For this review, take the finished solid that the model builds, in its own axes (mm). Face numbers are marked on the shaded views. A direction names the side the tool comes from. Round coordinates to 2 decimals unless told otherwise and drop trailing zeros. Write each loop counter-clockwise with the first axis right and the second up, starting at its lowest first coordinate (ties: lowest second). Pieces come first, ordered by that corner, then holes. Notation, with made-up numbers: M -6.75,-25 L 20.25,-25 A19 ccw 20.25,8 Z; hole C -31,-24 d3. An arc over 180 degrees is marked long. Answer in a Markdown table with one row per item.
```python
from build123d import *
from build123d.topology import SkipClean

# Parameters (mm, degrees)
ESQUISSE1_R             = 15
ESQUISSE1_R_2           = 10
BOSS_EXTRU_1_DEPTH      = 10
BOSS_EXTRU_2_START      = -10
ESQUISSE2_W             = 0.284758048
ESQUISSE2_H             = 1.526135502
BOSS_EXTRU_2_DEPTH      = 10
ESQUISSE3_R             = 1.5
ENL_V_MAT_EXTRU_1_DEPTH = 41.311288741


with BuildPart() as part:
    # Esquisse1 → Boss.-Extru.1 (new body)
    with BuildSketch(Plane.XY):
        Circle(ESQUISSE1_R)
        Circle(ESQUISSE1_R_2, mode=Mode.SUBTRACT)
    extrude(amount=BOSS_EXTRU_1_DEPTH)

    # Esquisse2 → Boss.-Extru.2 (add)
    with SkipClean():  # the faces are left unmerged after this step: merging them gives an invalid solid
        with BuildSketch(Plane.XY.offset(10).offset(BOSS_EXTRU_2_START)):
            with BuildLine():
                Line((15, 0), (15, -25))
                Line((15, -25), (5, -25))
                Line((5, -25), (5, -8.660254038))
                ThreePointArc((5, -8.660254038), (8.660254038, -5), (10, 0))
                Line((10, 0), (15, 0))
            make_face()
            with Locations((0, -15.401311239)):
                Rectangle(ESQUISSE2_W, ESQUISSE2_H)
            with BuildLine():
                Line((-10, 0), (-15, 0))
                Line((-15, 0), (-15, -25))
                Line((-15, -25), (-5, -25))
                Line((-5, -25), (-5, -8.660254038))
                ThreePointArc((-5, -8.660254038), (-8.660254038, -5), (-10, 0))
            make_face()
        extrude(amount=BOSS_EXTRU_2_DEPTH)

    # Esquisse3 → Enlèv. mat.-Extru.1 (cut, through all)
    with SkipClean():  # the faces are left unmerged after this step: merging them gives an invalid solid
        with BuildSketch(Plane.ZY.offset(15)):
            with Locations(Location((5, -21.5, 0), (0, 0, 270))):
                Circle(ESQUISSE3_R)
        extrude(amount=-ENL_V_MAT_EXTRU_1_DEPTH, mode=Mode.SUBTRACT)


solid = part.part
```
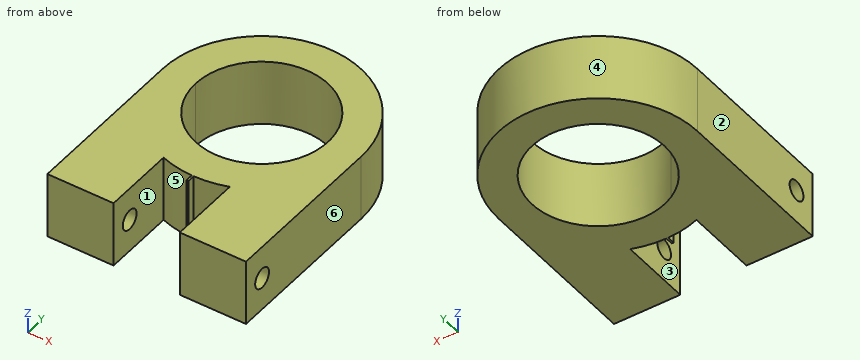
Q1. Insertion check: P1, Ø2, axis at x = -10.5, z = 4.5, coming from the +Y side; P2, Ø6, axis at y = 5, z = 5.5, coming from the -X side; P3, Ø1, axis at y = 4, z = 5.5, coming from the +X side. Each pin has a flat end and moves straight along its axis. Give the tip position at first contact, or say it passes through.
Found:
| item | result |
|---|---|
| P1 | y = 11.61 |
| P2 | x = -14.87 |
| P3 | x = 14.59 |
Q2. Mouldability with a two-part tool opening along X and no side actions: class the marked faces 3, 4, 5 and 6 as +X half, -X half, draft (parallel to the pull), parting line (faces both ways), or undercut.
Found:
| item | result |
|---|---|
| face 3 | undercut |
| face 4 | parting line |
| face 5 | undercut |
| face 6 | +X half |
Q3. Take a section at C-C (x = 7). State the section outline as (y, z) points.
Found:
| item | result |
|---|---|
| outline | M -25,0 L -7.14,0 L -7.14,10 L -25,10 Z; M 7.14,0 L 13.27,0 L 13.27,10 L 7.14,10 Z; hole C -21.5,5 d3 |
Q4. For probe 1 along Y at (x, z) = (0, 8.5); probe 2 along Z at (x, y) = (7.75, -21.5); probe 3 along X at (y, z) = (1.5, 1.25), list the stretches that pass through material, from the lowest coordinate up.
Found:
| item | result |
|---|---|
| probe 1 | -16.16 to -10, 10 to 15 |
| probe 2 | 0 to 3.5, 6.5 to 10 |
| probe 3 | -14.92 to -9.89, 9.89 to 14.92 |
Q5. Machinability: for the marked faces 1 and 2, which of the approach directions +Z, -Z, +X, -X, +Y, -Y give a long, thin tool a straight path to every point of the face, cutting with its end or side? Answer none if there is none.
Found:
| item | result |
|---|---|
| face 1 | +Z, -Z, -Y |
| face 2 | +Z, -Z, -X, +Y, -Y |
Q6. Take a section at D-D (z = 2). State the section outline as (x, y) points.
Found:
| item | result |
|---|---|
| outline | M -15,-25 L -5,-25 L -5,-14.14 A15 ccw -0.14,-15 L -0.14,-16.16 L 0.14,-16.16 L 0.14,-15 A15 ccw 5,-14.14 L 5,-25 L 15,-25 L 15,0 A15 ccw -15,0 Z; hole C 0,0 d20 |
Q7. Take a section at B-B (z = 5). State the section outline as (x, y) points, then the cut area to 3 significant figures.
Found:
| item | result |
|---|---|
| outline | M -15,-25 L -5,-25 L -5,-23 L -15,-23 Z; M -15,-20 L -5,-20 L -5,-14.14 A15 ccw -0.14,-15 L -0.14,-16.16 L 0.14,-16.16 L 0.14,-15 A15 ccw 5,-14.14 L 5,-20 L 15,-20 L 15,0 A15 ccw -15,0 Z; M 5,-25 L 15,-25 L 15,-23 L 5,-23 Z; hole C 0,0 d20 |
| area | 627 mm² |
Q8. Take a section at A-A (y = -21.5). State the section outline as (x, z) points.
Found:
| item | result |
|---|---|
| outline | M -15,0 L -5,0 L -5,3.5 L -15,3.5 Z; M -15,6.5 L -5,6.5 L -5,10 L -15,10 Z; M 5,0 L 15,0 L 15,3.5 L 5,3.5 Z; M 5,6.5 L 15,6.5 L 15,10 L 5,10 Z |
